```python
from build123d import *

# Parameters (mm, degrees)
F0_W     = 177.8
F0_H     = 29.5
F0_R     = 11
F0_H_2   = 22
F0_R_2   = 7.5
F0_H_3   = 21.5
F1_DEPTH = 5
F2_DEPTH = 60
F3_DEPTH = 70
F4_DEPTH = 70
F7_DEPTH = 80
F8_DEPTH = 90


with BuildPart() as f1:
    # F0 (on Top) → F1 (new body)
    with BuildSketch(Plane.XY):
        with Locations((0, 21.75)):
            Rectangle(F0_W, F0_H)
        with Locations((-73.9, 21.5)):
            Circle(F0_R, mode=Mode.SUBTRACT)
        with Locations((-49.3, 21.5)):
            Circle(F0_R, mode=Mode.SUBTRACT)
        with Locations((-24.7, 21.5)):
            Circle(F0_R, mode=Mode.SUBTRACT)
        with Locations((-0.1, 21.5)):
            Circle(F0_R, mode=Mode.SUBTRACT)
        with Locations((24.5, 21.5)):
            Circle(F0_R, mode=Mode.SUBTRACT)
        with Locations((49.1, 21.5)):
            Circle(F0_R, mode=Mode.SUBTRACT)
        with Locations((73.9, 21.5)):
            Circle(F0_R, mode=Mode.SUBTRACT)
        with Locations((0, -4)):
            Rectangle(F0_W, F0_H_2)
        with Locations((-61.6, -4)):
            Circle(F0_R_2, mode=Mode.SUBTRACT)
        with Locations((-37, -4)):
            Circle(F0_R_2, mode=Mode.SUBTRACT)
        with Locations((-12.4, -4)):
            Circle(F0_R_2, mode=Mode.SUBTRACT)
        with Locations((12.2, -4)):
            Circle(F0_R_2, mode=Mode.SUBTRACT)
        with Locations((36.8, -4)):
            Circle(F0_R_2, mode=Mode.SUBTRACT)
        with Locations((61.4, -4)):
            Circle(F0_R_2, mode=Mode.SUBTRACT)
        with Locations((0, -25.75)):
            Rectangle(F0_W, F0_H_3)
        with Locations((-61.6, -26)):
            Circle(F0_R_2, mode=Mode.SUBTRACT)
        with Locations((-37, -26)):
            Circle(F0_R_2, mode=Mode.SUBTRACT)
        with Locations((-12.4, -26)):
            Circle(F0_R_2, mode=Mode.SUBTRACT)
        with Locations((12.2, -26)):
            Circle(F0_R_2, mode=Mode.SUBTRACT)
        with Locations((36.8, -26)):
            Circle(F0_R_2, mode=Mode.SUBTRACT)
        with Locations((61.4, -26)):
            Circle(F0_R_2, mode=Mode.SUBTRACT)
        with Locations((-24.7, 21.5)):
            Circle(F0_R)
        with Locations((-49.3, 21.5)):
            Circle(F0_R)
        with Locations((-73.9, 21.5)):
            Circle(F0_R)
        with Locations((24.5, 21.5)):
            Circle(F0_R)
        with Locations((73.9, 21.5)):
            Circle(F0_R)
        with Locations((49.1, 21.5)):
            Circle(F0_R)
        with Locations((-0.1, 21.5)):
            Circle(F0_R)
        with Locations((36.8, -4)):
            Circle(F0_R_2)
        with Locations((12.2, -26)):
            Circle(F0_R_2)
        with Locations((-12.4, -4)):
            Circle(F0_R_2)
        with Locations((-12.4, -26)):
            Circle(F0_R_2)
        with Locations((12.2, -4)):
            Circle(F0_R_2)
        with Locations((61.4, -4)):
            Circle(F0_R_2)
        with Locations((-37, -4)):
            Circle(F0_R_2)
        with Locations((-61.6, -4)):
            Circle(F0_R_2)
        with Locations((-37, -26)):
            Circle(F0_R_2)
        with Locations((-61.6, -26)):
            Circle(F0_R_2)
        with Locations((61.4, -26)):
            Circle(F0_R_2)
        with Locations((36.8, -26)):
            Circle(F0_R_2)
    extrude(amount=-F1_DEPTH)

    # F0 (on Top) → F2 (join)
    with BuildSketch(Plane.XY):
        with Locations((0, -25.75)):
            Rectangle(F0_W, F0_H_3)
        with Locations((-61.6, -26)):
            Circle(F0_R_2, mode=Mode.SUBTRACT)
        with Locations((-37, -26)):
            Circle(F0_R_2, mode=Mode.SUBTRACT)
        with Locations((-12.4, -26)):
            Circle(F0_R_2, mode=Mode.SUBTRACT)
        with Locations((12.2, -26)):
            Circle(F0_R_2, mode=Mode.SUBTRACT)
        with Locations((36.8, -26)):
            Circle(F0_R_2, mode=Mode.SUBTRACT)
        with Locations((61.4, -26)):
            Circle(F0_R_2, mode=Mode.SUBTRACT)
    extrude(amount=F2_DEPTH)

    # F0 (on Top) → F3 (join)
    with BuildSketch(Plane.XY):
        with Locations((0, -4)):
            Rectangle(F0_W, F0_H_2)
        with Locations((-61.6, -4)):
            Circle(F0_R_2, mode=Mode.SUBTRACT)
        with Locations((-37, -4)):
            Circle(F0_R_2, mode=Mode.SUBTRACT)
        with Locations((-12.4, -4)):
            Circle(F0_R_2, mode=Mode.SUBTRACT)
        with Locations((12.2, -4)):
            Circle(F0_R_2, mode=Mode.SUBTRACT)
        with Locations((36.8, -4)):
            Circle(F0_R_2, mode=Mode.SUBTRACT)
        with Locations((61.4, -4)):
            Circle(F0_R_2, mode=Mode.SUBTRACT)
        with Locations((-61.6, -4)):
            Circle(F0_R_2)
        with Locations((-37, -4)):
            Circle(F0_R_2)
        with Locations((-12.4, -4)):
            Circle(F0_R_2)
        with Locations((12.2, -4)):
            Circle(F0_R_2)
        with Locations((36.8, -4)):
            Circle(F0_R_2)
        with Locations((61.4, -4)):
            Circle(F0_R_2)
    extrude(amount=F3_DEPTH)


with BuildPart() as f4:
    # F0 (on Top) → F4 (new body)
    with BuildSketch(Plane.XY):
        with Locations((-61.6, -4)):
            Circle(F0_R_2)
    extrude(amount=F4_DEPTH)


with BuildPart() as f4b:
    # F0 (on Top) → F4, piece 2 (new body)
    with BuildSketch(Plane.XY):
        with Locations((-37, -4)):
            Circle(F0_R_2)
    extrude(amount=F4_DEPTH)


with BuildPart() as f4c:
    # F0 (on Top) → F4, piece 3 (new body)
    with BuildSketch(Plane.XY):
        with Locations((-12.4, -4)):
            Circle(F0_R_2)
    extrude(amount=F4_DEPTH)


with BuildPart() as f4d:
    # F0 (on Top) → F4, piece 4 (new body)
    with BuildSketch(Plane.XY):
        with Locations((12.2, -4)):
            Circle(F0_R_2)
    extrude(amount=F4_DEPTH)


with BuildPart() as f4e:
    # F0 (on Top) → F4, piece 5 (new body)
    with BuildSketch(Plane.XY):
        with Locations((36.8, -4)):
            Circle(F0_R_2)
    extrude(amount=F4_DEPTH)


with BuildPart() as f4f:
    # F0 (on Top) → F4, piece 6 (new body)
    with BuildSketch(Plane.XY):
        with Locations((61.4, -4)):
            Circle(F0_R_2)
    extrude(amount=F4_DEPTH)


with BuildPart() as f4_1:
    # F5: moved
    add(f4.part.moved(Location((0, 0, 10))))


with BuildPart() as f4b_1:
    # F5: moved
    add(f4b.part.moved(Location((0, 0, 10))))


with BuildPart() as f4c_1:
    # F5: moved
    add(f4c.part.moved(Location((0, 0, 10))))


with BuildPart() as f4d_1:
    # F5: moved
    add(f4d.part.moved(Location((0, 0, 10))))


with BuildPart() as f4e_1:
    # F5: moved
    add(f4e.part.moved(Location((0, 0, 10))))


with BuildPart() as f4f_1:
    # F5: moved
    add(f4f.part.moved(Location((0, 0, 10))))


with BuildPart() as f1_1:
    add(f1.part)

    # F6: cut F4, F4b, F4c, F4d, F4e, F4f
    add(f4_1.part, mode=Mode.SUBTRACT)
    add(f4b_1.part, mode=Mode.SUBTRACT)
    add(f4c_1.part, mode=Mode.SUBTRACT)
    add(f4d_1.part, mode=Mode.SUBTRACT)
    add(f4e_1.part, mode=Mode.SUBTRACT)
    add(f4f_1.part, mode=Mode.SUBTRACT)

    # F0 (on Top) → F7 (join)
    with BuildSketch(Plane.XY):
        with Locations((0, 21.75)):
            Rectangle(F0_W, F0_H)
        with Locations((-73.9, 21.5)):
            Circle(F0_R, mode=Mode.SUBTRACT)
        with Locations((-49.3, 21.5)):
            Circle(F0_R, mode=Mode.SUBTRACT)
        with Locations((-24.7, 21.5)):
            Circle(F0_R, mode=Mode.SUBTRACT)
        with Locations((-0.1, 21.5)):
            Circle(F0_R, mode=Mode.SUBTRACT)
        with Locations((24.5, 21.5)):
            Circle(F0_R, mode=Mode.SUBTRACT)
        with Locations((49.1, 21.5)):
            Circle(F0_R, mode=Mode.SUBTRACT)
        with Locations((73.9, 21.5)):
            Circle(F0_R, mode=Mode.SUBTRACT)
        with Locations((-73.9, 21.5)):
            Circle(F0_R)
        with Locations((-49.3, 21.5)):
            Circle(F0_R)
        with Locations((-24.7, 21.5)):
            Circle(F0_R)
        with Locations((-0.1, 21.5)):
            Circle(F0_R)
        with Locations((24.5, 21.5)):
            Circle(F0_R)
        with Locations((49.1, 21.5)):
            Circle(F0_R)
        with Locations((73.9, 21.5)):
            Circle(F0_R)
    extrude(amount=F7_DEPTH)


with BuildPart() as f8:
    # F0 (on Top) → F8 (new body)
    with BuildSketch(Plane.XY):
        with Locations((-73.9, 21.5)):
            Circle(F0_R)
    extrude(amount=F8_DEPTH)


with BuildPart() as f8b:
    # F0 (on Top) → F8, piece 2 (new body)
    with BuildSketch(Plane.XY):
        with Locations((-49.3, 21.5)):
            Circle(F0_R)
    extrude(amount=F8_DEPTH)


with BuildPart() as f8c:
    # F0 (on Top) → F8, piece 3 (new body)
    with BuildSketch(Plane.XY):
        with Locations((-24.7, 21.5)):
            Circle(F0_R)
    extrude(amount=F8_DEPTH)


with BuildPart() as f8d:
    # F0 (on Top) → F8, piece 4 (new body)
    with BuildSketch(Plane.XY):
        with Locations((-0.1, 21.5)):
            Circle(F0_R)
    extrude(amount=F8_DEPTH)


with BuildPart() as f8e:
    # F0 (on Top) → F8, piece 5 (new body)
    with BuildSketch(Plane.XY):
        with Locations((24.5, 21.5)):
            Circle(F0_R)
    extrude(amount=F8_DEPTH)


with BuildPart() as f8f:
    # F0 (on Top) → F8, piece 6 (new body)
    with BuildSketch(Plane.XY):
        with Locations((49.1, 21.5)):
            Circle(F0_R)
    extrude(amount=F8_DEPTH)


with BuildPart() as f8g:
    # F0 (on Top) → F8, piece 7 (new body)
    with BuildSketch(Plane.XY):
        with Locations((73.9, 21.5)):
            Circle(F0_R)
    extrude(amount=F8_DEPTH)


with BuildPart() as f8_1:
    # F9: moved
    add(f8.part.moved(Location((0, 0, 20))))


with BuildPart() as f8g_1:
    # F9: moved
    add(f8g.part.moved(Location((0, 0, 20))))


with BuildPart() as f8b_1:
    # F9: moved
    add(f8b.part.moved(Location((0, 0, 20))))


with BuildPart() as f8c_1:
    # F9: moved
    add(f8c.part.moved(Location((0, 0, 20))))


with BuildPart() as f8d_1:
    # F9: moved
    add(f8d.part.moved(Location((0, 0, 20))))


with BuildPart() as f8e_1:
    # F9: moved
    add(f8e.part.moved(Location((0, 0, 20))))


with BuildPart() as f8f_1:
    # F9: moved
    add(f8f.part.moved(Location((0, 0, 20))))


with BuildPart() as f1_2:
    add(f1_1.part)

    # F10: cut F8, F8g, F8b, F8c, F8d, F8e, F8f
    add(f8_1.part, mode=Mode.SUBTRACT)
    add(f8g_1.part, mode=Mode.SUBTRACT)
    add(f8b_1.part, mode=Mode.SUBTRACT)
    add(f8c_1.part, mode=Mode.SUBTRACT)
    add(f8d_1.part, mode=Mode.SUBTRACT)
    add(f8e_1.part, mode=Mode.SUBTRACT)
    add(f8f_1.part, mode=Mode.SUBTRACT)


solid = f1_2.part
```
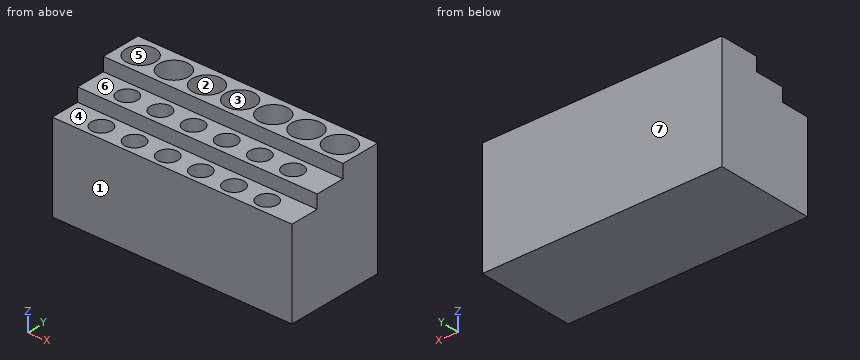
Here's how the part is built. I have some questions about the finished solid (model axes, mm). Face numbers are marked on the shaded views. A direction names the side the tool comes from. Round coordinates to 2 decimals unless told otherwise and drop trailing zeros. Order: outer loops, then holes, each group sorted by start corner. A loop starts at its lowest first (then second) coordinate and runs counter-clockwise, first axis right, second up. Notation, with made-up numbers: M 64.25,-0.75 L 92.25,-0.75 A13 cw 92.25,17.25 Z; hole C 41,44 d5. An arc over 180 degrees is marked long. Answer in a Markdown table with one row per item.
Item 1: For the marked faces 5, 6 and 7, which set-ups out of +Z, -Z, +X, -X, +Y, -Y let a thin tool reach every point of the face, with its end or its side?
A:
| item | result |
|---|---|
| face 5 | +Z |
| face 6 | +Z, +X, -X, -Y |
| face 7 | +Z, -Z, +X, -X, +Y |
Item 2: I'm going to push flat-ended pins straight in: pin 1 (12 mm diameter, centred on x = -37, y = -26, fed in from +Z); pin 2 (4.5 mm diameter, centred on x = -36.5, y = -4, fed in from +Z); pin 3 (12 mm diameter, centred on x = 35, y = -5.5, fed in from +Z). Where does each tip first touch, or does it pass through?
A:
| item | result |
|---|---|
| pin 1 | stops at z = 0 |
| pin 2 | stops at z = 10 |
| pin 3 | stops at z = 70 |
Item 3: Imagine slicing it at C-C, the plane x = 49.1. Write out the boundary of the cut face in (y, z).
A:
| item | result |
|---|---|
| outline | M -36.5,-5 L 36.5,-5 L 36.5,80 L 32.5,80 L 32.5,20 L 10.5,20 L 10.5,80 L 7,80 L 7,70 L -15,70 L -15,60 L -36.5,60 Z |
Item 4: If I drill on L1, parallel to Y at x = -12.4, z = 25.5; L2, parallel to Y at x = -56, z = 48.5; L3, parallel to Y at x = 73.9, z = 55.5, over which ranges is the centre line in solid material (lowest first)? Write a range as from..to.
A:
| item | result |
|---|---|
| L1 | y = -36.5..-33.5, -18.5..-11.5, 3.5..36.5 |
| L2 | y = -36.5..-30.99, -21.01..-8.99, 0.99..12.78, 30.22..36.5 |
| L3 | y = -36.5..10.5, 32.5..36.5 |
Item 5: Imagine slicing it at D-D, the plane y = -4. Write out the boundary of the cut face in (x, z), and give its area (4 significant figures).
A:
| item | result |
|---|---|
| outline | M -88.9,-5 L 88.9,-5 L 88.9,70 L 68.9,70 L 68.9,10 L 53.9,10 L 53.9,70 L 44.3,70 L 44.3,10 L 29.3,10 L 29.3,70 L 19.7,70 L 19.7,10 L 4.7,10 L 4.7,70 L -4.9,70 L -4.9,10 L -19.9,10 L -19.9,70 L -29.5,70 L -29.5,10 L -44.5,10 L -44.5,70 L -54.1,70 L -54.1,10 L -69.1,10 L -69.1,70 L -88.9,70 Z |
| area | 7,935 mm2 |
Item 6: Thinking about a two-plate mould opening in Y: for the marked faces 1, 2, 3 and 4, which applies, +Y half, -Y half, draft (parallel to the pull), parting line (faces both ways), or undercut?
A:
| item | result |
|---|---|
| face 1 | -Y half |
| face 2 | undercut |
| face 3 | undercut |
| face 4 | draft |
Item 7: Imagine slicing it at A-A, the plane z = 64.5. State how many separate pieces and enclosed holes the cut face has, and give its area (3 significant figures).
A:
| item | result |
|---|---|
| separate pieces | 1 |
| enclosed holes | 13 |
| area | 5,440 mm2 |
